Read the model definition and answer for the solid it produces. Units are mm, in the model's axes. A direction names the side the tool comes from. Give positions to 0.01 mm unless a question says otherwise; leave off trailing zeros. Loops run counter-clockwise (first coordinate to the right, second up) from the corner with the lowest first, then second, coordinate; pieces in that order, holes last. Notation, with made-up numbers: (-22.5, 37.5) - (-13.5, 37.5) arc R20 ccw to (-13.5, 71.5) - close; hole circle Ø4 at (1.5, -9.75). An arc over 180 degrees is marked (long way). Put each result on its own line as item: value. Start each with the question number.
1. For a pull along Z with two mould halves and no side action, classify faces 1 (the cylindrical face through (0.33, 4.198, -7.493)), 2 (the flat face through (0, 0, 0)), 3 (the flat face through (1, 12, 0)) as released by +Z, released by -Z, zero draft, split by the parting line, or undercut.
2. A cutting plane is placed at C-C, the plane y = 13.5. Determine the outline of the cut face in (x, z), plus the area to 3 significant figures.
3. Consider L1, parallel to X at y = 7.75, z = 0; L2, parallel to X at y = 9, z = 0; L3, parallel to Y at x = -6.25, z = -2.75. Determine where each line is inside the solid, lowest interval first. Write a range as from..to.
4. For faces 4 (the cylindrical face through (7.25, 13.52, -0.07)), 5 (the flat face through (-7, 8, 0)), 6 (the flat face through (8, 8, 0)), determine the directions among +Z, -Z, +X, -X, +Y, -Y from which every point of the face is accessible in a straight line to the end or side of a thin tool.
5. A cutting plane is placed at B-B, the plane y = 5.75. Determine the outline of the cut face in (x, z), plus the area to 3 significant figures.
6. Given pin 1 Ø6.5 at (x, z) = (4, 0.5) entering from -Y; pin 2 Ø5 at (y, z) = (12, -1.5) entering from -X; pin 3 Ø4 at (x, y) = (5, 12.5) entering from -Z; pin 4 Ø0.9 at (x, y) = (0, 14) entering from -Z, each flat-ended and moving along its own axis, determine where each tip first touches the part or whether it passes through.
7. A cutting plane is placed at A-A, the plane z = 0. Determine the outline of the cut face in (x, y), plus the area to 3 significant figures.
```python
from build123d import *

# Parameters (mm, degrees)
SKETCH1_R           = 7.5
BOSS_EXTRUDE1_DEPTH = 8
SKETCH2_R           = 7.5
BOSS_EXTRUDE2_DEPTH = 7
SKETCH3_R           = 1.5
CUT_EXTRUDE1_DEPTH  = 19.801595677
CUT_EXTRUDE3_DEPTH  = 3
CHAMFER1_SIZE       = 0.5


with BuildPart() as part:
    # Sketch1 → Boss-Extrude1 (new body)
    with BuildSketch(Plane(origin=(0, 0, 0), x_dir=(1, 0, 0), z_dir=(0, 1, 0))):
        with Locations(Location((0, 0, 0), (0, 0, 270))):
            Circle(SKETCH1_R)
    extrude(amount=BOSS_EXTRUDE1_DEPTH)

    # Sketch2 → Boss-Extrude2 (add)
    with BuildSketch(Plane(origin=(0, 8, 0), x_dir=(1, 0, 0), z_dir=(0, 1, 0))):
        with Locations(Location((1, 0, 0), (0, 0, 93.822553729))):
            Circle(SKETCH2_R)
    extrude(amount=BOSS_EXTRUDE2_DEPTH)

    # Sketch3 → Cut-Extrude1 (cut, through all)
    with BuildSketch(Plane(origin=(0, 15, 0), x_dir=(1, 0, 0), z_dir=(0, 1, 0))):
        with Locations(Location((-2.25, 0, 0), (0, 0, 270))):
            Circle(SKETCH3_R)
        with Locations(Location((4.25, 0, 0), (0, 0, 270))):
            Circle(SKETCH3_R)
    extrude(amount=-CUT_EXTRUDE1_DEPTH, mode=Mode.SUBTRACT)

    # Sketch5 → Cut-Extrude3 (cut)
    with BuildSketch(Plane(origin=(0, 15, 0), x_dir=(1, 0, 0), z_dir=(0, 1, 0))):
        with BuildLine():
            Line((-2.25, 3), (4.25, 3))
            ThreePointArc((4.25, 3), (7.25, 0), (4.25, -3))
            Line((4.25, -3), (-2.25, -3))
            ThreePointArc((-2.25, -3), (-5.25, 0), (-2.25, 3))
        make_face()
    extrude(amount=-CUT_EXTRUDE3_DEPTH, mode=Mode.SUBTRACT)

    # Chamfer1
    chamfer1_edges = [part.edges().sort_by_distance(p)[0] for p in [
        (0, 0, -7.5),
        (1.5, 15, 7.483314774),
    ]]
    chamfer(chamfer1_edges, length=CHAMFER1_SIZE)


solid = part.part
```
Return value:
1. face 1: split by the parting line
1. face 2: zero draft
1. face 3: undercut
2. outline: circle Ø15 at (1, 0); hole (-2.25, -3) - (4.25, -3) arc R3 ccw to (4.25, 3) - (-2.25, 3) arc R3 ccw to start
2. area: 109 mm2
3. L1: x = -7.5..-3.75, -0.75..2.75, 5.75..7.5
3. L2: x = -6.5..-3.75, -0.75..2.75, 5.75..8.5
3. L3: y = 0..8
4. face 4: +Y
4. face 5: -X, +Y
4. face 6: +X, -Y
5. outline: circle Ø15 at (0, 0); hole circle Ø3 at (-2.25, 0); hole circle Ø3 at (4.25, 0)
5. area: 163 mm2
6. pin 1: stops at y = 0
6. pin 2: stops at x = -6.5
6. pin 3: stops at z = -7.23
6. pin 4: stops at z = -7.48
7. outline: (-7.5, 0.5) - (-7, 0) - (-3.75, 0) - (-3.75, 12) - (-5.25, 12) - (-5.25, 15) - (-6, 15) - (-6.5, 14.5) - (-6.5, 8) - (-7.5, 8) - close; (-0.75, 0) - (2.75, 0) - (2.75, 12) - (-0.75, 12) - close; (5.75, 0) - (7, 0) - (7.5, 0.5) - (7.5, 8) - (8.5, 8) - (8.5, 14.5) - (8, 15) - (7.25, 15) - (7.25, 12) - (5.75, 12) - close
7. area: 115 mm2
